Can you work these out from the model? Positions are in its coordinate system, mm. A direction names the side the tool comes from. Coordinates: 2 decimals unless noted, no trailing zeros. Loops run counter-clockwise (first coordinate to the right, second up) from the corner with the lowest first, then second, coordinate; pieces in that order, holes last. Notation, with made-up numbers: M -36.75,53.25 L 4.25,53.25 A36 cw 4.25,87.25 Z; hole C -28.5,85 d5. An arc over 180 degrees is marked long. Answer as a JSON object with one key per item and string values. Group by question number.
Item 1: Suppose I cut it at A-A (x = 0). Write out the boundary of the cut face in (y, z).
Item 2: If I drill on line 1 (Y direction, x = 4.5, z = 8.85); line 2 (Z direction, x = -1.5, y = 1.75); line 3 (Z direction, x = 1.75, y = 0.25), over which ranges is the centre line in solid material (lowest first)?
Item 3: Which directions (+Z, -Z, +X, -X, +Y, -Y) give clear straight access to the entire face, cutting with the end or side of a thin tool? Please do faces 4 (the cylindrical face through (4.5, 2.96, 4.06)), 5 (the flat face through (0, 0, -15)), 6 (the cylindrical face through (0, -2, 37)).
Item 4: I'm going to push flat-ended pins straight in: pin 1 Ø2 at (y, z) = (-1, 44.5) entering from -X; pin 2 Ø4 at (x, z) = (-3.5, 41.5) entering from -Y; pin 3 Ø0.8 at (x, y) = (-4.5, -0.14) entering from +Z. Where does each tip first touch, or does it pass through?
Item 5: Suppose I cut it at B-B (z = 40). Write out the boundary of the cut face in (x, y).
Item 6: We'd pull the mould along Y, two halves only. Please class faces 1 (the cylindrical face through (-3.876, -0.112, 8.493)), 2 (the flat face through (0, -5, -7)), 3 (the flat face through (6, 0, -7)): +Y half, -Y half, draft (parallel to the pull), parting line (faces both ways), or undercut.
```python
from build123d import *

# Parameters (mm, degrees)
SKETCH2_W               = 12
SKETCH2_H               = 10
BOSS_EXTRUDE1_DEPTH     = 15
SKETCH3_W               = 12
SKETCH3_H               = 10
BOSS_EXTRUDE2_DEPTH     = 1
SKETCH4_R               = 2
BOSS_EXTRUDE3_DEPTH     = 56
BOSS_EXTRUDE4_REACH     = 59.533
SKETCH5_R               = 1
M1_6_TAPPED_HOLE1_D     = 1.25
M1_6_TAPPED_HOLE1_DEPTH = 4.25
M1_6_TAPPED_HOLE1_TIP   = 0.375537887


with BuildPart() as part:
    # Sketch2 → Boss-Extrude1 (new body)
    with BuildSketch(Plane.XY):
        Rectangle(SKETCH2_W, SKETCH2_H)
    extrude(amount=-BOSS_EXTRUDE1_DEPTH)

    # Sketch5 → Boss-Extrude4 (add, up to next)
    with BuildSketch(Plane(origin=(0, 0, 8), x_dir=(-1, 0, 0), z_dir=(0, 0, -1)), mode=Mode.PRIVATE) as boss_extrude4_sk1:
        with Locations((-3.5, 2.916666667)):
            Circle(SKETCH5_R)
    boss_extrude4_tool1 = extrude(boss_extrude4_sk1.sketch, amount=BOSS_EXTRUDE4_REACH, mode=Mode.PRIVATE) - part.part
    # Sketch5 → Boss-Extrude4 (add, up to next)
    with BuildSketch(Plane(origin=(0, 0, 8), x_dir=(-1, 0, 0), z_dir=(0, 0, -1)), mode=Mode.PRIVATE) as boss_extrude4_sk2:
        with Locations((3.5, -2.916666667)):
            Circle(SKETCH5_R)
    boss_extrude4_tool2 = extrude(boss_extrude4_sk2.sketch, amount=BOSS_EXTRUDE4_REACH, mode=Mode.PRIVATE) - part.part


with BuildPart() as body_2:
    # Sketch3 → Boss-Extrude2 (new body)
    with BuildSketch(Plane.XY.offset(9)):
        Rectangle(SKETCH3_W, SKETCH3_H)
    extrude(amount=-BOSS_EXTRUDE2_DEPTH)

    # Sketch4 → Boss-Extrude3 (add)
    with BuildSketch(Plane.XY.offset(9)):
        Circle(SKETCH4_R)
    extrude(amount=BOSS_EXTRUDE3_DEPTH)


with BuildPart() as part_1:
    add(part.part)

    add(body_2.part)  # Boss-Extrude4 merges body 2
    add(boss_extrude4_tool1.solids().sort_by_distance((3.5, 2.916667, 8))[0])
    add(boss_extrude4_tool2.solids().sort_by_distance((-3.5, -2.916667, 8))[0])

    # M1.6 Tapped Hole1
    with Locations(Plane.XY.offset(9)):
        with Locations((-4.5, -0.139522792), (4.5, -0.139522792)):
            Hole(M1_6_TAPPED_HOLE1_D / 2, depth=M1_6_TAPPED_HOLE1_DEPTH)
            with Locations((0, 0, -(M1_6_TAPPED_HOLE1_DEPTH + M1_6_TAPPED_HOLE1_TIP / 2))):  # 118° drill point
                Cone(0, M1_6_TAPPED_HOLE1_D / 2, M1_6_TAPPED_HOLE1_TIP, mode=Mode.SUBTRACT)


solid = part_1.part
```
From the geometry:
{
 "1": {"outline": "M -5,-15 L 5,-15 L 5,0 L -5,0 Z; M -5,8 L 5,8 L 5,9 L 2,9 L 2,65 L -2,65 L -2,9 L -5,9 Z"},
 "2": {"line 1": "-5 to -0.76, 0.49 to 5", "line 2": "-15 to 0, 8 to 9", "line 3": "-15 to 0, 8 to 65"},
 "3": {"face 4": "none", "face 5": "-Z, +X, -X, +Y, -Y", "face 6": "+Z"},
 "4": {"pin 1": "x = -2", "pin 2": "y = -1.32", "pin 3": "z = 0"},
 "5": {"outline": "C 0,0 d4"},
 "6": {"face 1": "undercut", "face 2": "-Y half", "face 3": "draft"}
}
